Input: part model. Units: mm. Frame: model coordinates. A direction names the side the tool comes from. Coordinates: 2 decimals unless noted, no trailing zeros. Write each loop counter-clockwise with the first axis right and the second up, starting at its lowest first coordinate (ties: lowest second). Pieces come first, ordered by that corner, then holes. Notation, with made-up numbers: (-32.5, -33) -> (8.5, -33) arc R33 ccw to (8.5, 2) -> close; hole circle Ø9 at (56.5, 80). An arc over 180 degrees is marked (long way). Use one line per item in the form item = value. Start each with the question number.
(1) Ray query, line 1 along Y through (x, z) = (7, 20); line 2 along Y through (x, z) = (4.5, 8); line 3 along X through (y, z) = (15, 14). Return the intervals inside material, ascending.
(2) First-contact query: pin 1 (12 mm diameter, centred on x = 1.5, z = 24.5, fed in from +Y); pin 2 (10 mm diameter, centred on y = 29.5, z = 19.5, fed in from +X); pin 3 (16 mm diameter, centred on x = 7, y = 14, fed in from +Z); pin 4 (8 mm diameter, centred on x = 8.5, z = 23.5, fed in from -Y). Flat tips, straight axial feed; report the tip coordinate or a pass-through.
(3) Cut plane B-B on z = 19.5. Return the cut outline in (x, y).
(4) Set-up query: faces 4 (the face through (14, 0, 21)), 5 (the face through (-7, 16, 21)), 6 (the face through (3, 32, 21)). Return all of +Z, -Z, +X, -X, +Y, -Y with unobstructed straight access to the full face (end or side cutting, diameter ignored); none if empty.
(5) Pull-direction query (X, two-part tool) for faces 1 (the face through (34, 16, 0)), 2 (the face through (35.397, -12.22, 21.199)), 3 (the face through (15.45, 30.51, 21.2)); classes: released by +X, released by -X, zero draft, split by the parting line, or undercut.
(6) Cut plane C-C on x = 56. Return the cut outline in (y, z), plus the area to 3 significant figures.
(7) Cut plane A-A on y = 16. Return the cut outline in (x, z).
(8) Cut plane D-D on y = 26.5. Return the cut outline in (x, z), plus the area to 3 significant figures.
```python
from build123d import *

# Parameters (mm, degrees)
SKETCH1_R           = 7
BOSS_EXTRUDE1_DEPTH = 43


with BuildPart() as part:
    # Sketch1 → Boss-Extrude1 (new body)
    with BuildSketch(Plane.XY):
        with BuildLine():
            Line((0, 0), (-7, 7))
            Line((-7, 7), (-7, 25))
            Line((-7, 25), (0, 32))
            Line((0, 32), (7, 32))
            Line((7, 32), (24.131881406, 28.979187078))
            ThreePointArc((24.131881406, 28.979187078), (35.36077259, 30.424329605), (43.774193548, 38))
            Line((43.774193548, 38), (67.084538376, 38))
            Line((67.084538376, 38), (72.774193548, 33))
            Line((72.774193548, 33), (74, 14))
            Line((74, 14), (45, -19))
            Line((45, -19), (39.788067397, -19))
            ThreePointArc((39.788067397, -19), (35.3490952, -12.115672061), (33.012264997, -4.264705882))
            ThreePointArc((33.012264997, -4.264705882), (31.331862036, -1.213413768), (28.066626255, 0))
            Line((28.066626255, 0), (0, 0))
        make_face()
        with Locations((7, 14)):
            Circle(SKETCH1_R, mode=Mode.SUBTRACT)
    extrude(amount=BOSS_EXTRUDE1_DEPTH)


solid = part.part
```
Values:
q1.line_1 = 0 to 7, 21 to 32
q1.line_2 = 0 to 7.46, 20.54 to 32
q1.line_3 = -7 to 0.07, 13.93 to 73.94
q2.pin_1 = 32
q2.pin_2 = 73.32
q2.pin_3 = 43
q2.pin_4 = 0
q3.outline = (-7, 7) -> (0, 0) -> (28.07, 0) arc R5 cw to (33.01, -4.26) arc R29 ccw to (39.79, -19) -> (45, -19) -> (74, 14) -> (72.77, 33) -> (67.08, 38) -> (43.77, 38) arc R19 cw to (24.13, 28.98) -> (7, 32) -> (0, 32) -> (-7, 25) -> close; hole circle Ø14 at (7, 14)
q4.face_4 = +Z, -Z, -X, -Y
q4.face_5 = +Z, -Z, -X, +Y, -Y
q4.face_6 = +Z, -Z, -X, +Y
q5.face_1 = zero draft
q5.face_2 = released by -X
q5.face_3 = undercut
q6.outline = (-6.48, 0) -> (38, 0) -> (38, 43) -> (-6.48, 43) -> close
q6.area = 1,910 mm2
q7.outline = (-7, 0) -> (0.29, 0) -> (0.29, 43) -> (-7, 43) -> close; (13.71, 0) -> (73.87, 0) -> (73.87, 43) -> (13.71, 43) -> close
q8.outline = (-5.5, 0) -> (73.19, 0) -> (73.19, 43) -> (-5.5, 43) -> close
q8.area = 3,380 mm2
